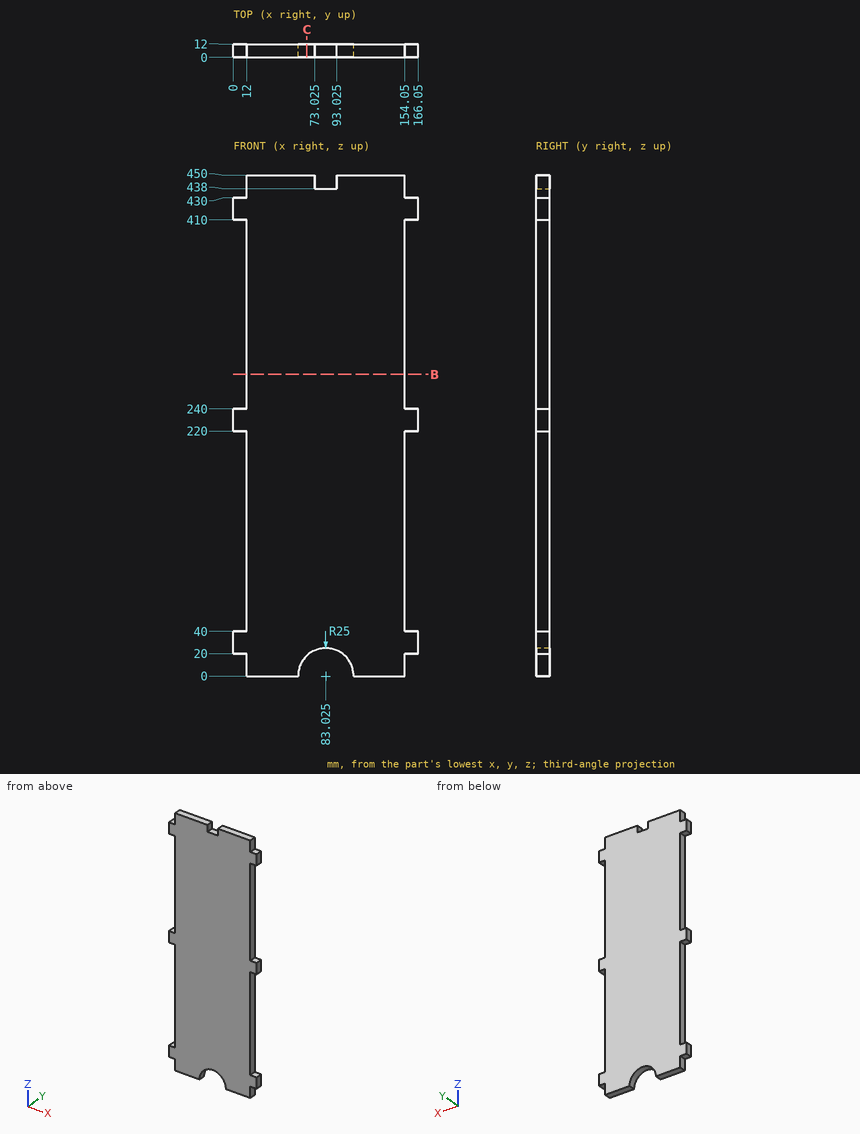
The figure shows three views and two pictorial views of one solid part (mm, origin at its lowest corner). Answer the questions. Give positions to 0.01 mm unless a question says otherwise; leave off trailing zeros. Write each loop counter-clockwise with the first axis right and the second up, starting at its lowest first coordinate (ties: lowest second). Pieces come first, ordered by that corner, then holes.
Q1. Given pin 1 (6 mm diameter, centred on y = 8, z = 7.5, fed in from +X); pin 2 (3 mm diameter, centred on y = 10.5, z = 192.5, fed in from -X); pin 3 (3.5 mm diameter, centred on x = 160.5, y = 7.5, fed in from +Z), each flat-ended and moving along its own axis, determine where each tip first touches the part or whether it passes through.
Answer:
pin 1: stops at x = 154.05
pin 2: stops at x = 12
pin 3: stops at z = 430
Q2. Straight lines are drawn through the part: L1, parallel to X at y = 4.75, z = 250; L2, parallel to Z at x = 68, y = 3.25; L3, parallel to Z at x = 95, y = 2. For each, find the intervals that lie inside material, in ascending order.
Answer:
L1: x = 12 to 154.05
L2: z = 19.98 to 450
L3: z = 21.95 to 450
Q3. The part is cut by section C-C on x = 66. Give the vertices of the cut face in (y, z).
Answer:
outline: (0, 18.31) - (12, 18.31) - (12, 450) - (0, 450) - close
Q4. The part is cut by section B-B on z = 271. Give the vertices of the cut face in (x, y), and give its area (3 significant figures).
Answer:
outline: (12, 0) - (154.05, 0) - (154.05, 12) - (12, 12) - close
area: 1,700 mm2
